```python
from build123d import *
from build123d.topology import SkipClean

# Parameters (mm, degrees)
EXTRUDE_1_DEPTH          = 48.25
EXTRUDE_1_DEPTH_BACK     = 48.25
EXTRUDE_2_DEPTH          = 3.75
EXTRUDE_2_DEPTH_BACK     = 3.75
SKETCH_2_R               = 7.5
SKETCH_2_R_2             = 5
CUT_EXTRUDE_1_DEPTH      = 3.75
CUT_EXTRUDE_1_DEPTH_BACK = 3.75
SKETCH_3_R               = 5
EXTRUDE_3_DEPTH          = 11.5
EXTRUDE_3_DEPTH_BACK     = 3.75
SKETCH_4_R               = 10
CUT_EXTRUDE_4_DEPTH      = 2
SKETCH_9_R               = 7.5
CUT_EXTRUDE_5_DEPTH      = 5
EXTRUDE_START            = 9
SKETCH_10_R              = 10
SKETCH_10_R_2            = 8.5
EXTRUDE_5_DEPTH          = 9
SKETCH_11_R              = 2.95
CUT_EXTRUDE_6_DEPTH      = 2
SKETCH_12_R              = 5.5
CUT_EXTRUDE_7_DEPTH      = 6
CUT_EXTRUDE_START        = -6
SKETCH_13_R              = 2.95
CUT_EXTRUDE_8_DEPTH      = 6


with BuildPart() as part:
    # Sketch 1 → Extrude 1 (new, two sides: drawn at the far end of the back side and taken through both)
    with BuildSketch(Plane(origin=(0, 0, 0), x_dir=(0, 0, -1), z_dir=(1, 0, 0)).offset(-EXTRUDE_1_DEPTH_BACK)):
        Polygon((3.75, 0), (3.75, 7.5), (-3.75, 7.5), (-3.75, -7.5), (3.75, -7.5), align=None)
    extrude(amount=EXTRUDE_1_DEPTH + EXTRUDE_1_DEPTH_BACK)

    # Sketch 2 → Extrude 2 (add, two sides: drawn at the far end of the back side and taken through both)
    with BuildSketch(Plane.XY.offset(-EXTRUDE_2_DEPTH_BACK)):
        with Locations((-48.25, 0)):
            Circle(SKETCH_2_R)
        with Locations((-48.25, 0)):
            Circle(SKETCH_2_R_2, mode=Mode.SUBTRACT)
    extrude(amount=EXTRUDE_2_DEPTH + EXTRUDE_2_DEPTH_BACK)

    # Sketch 3 → Cut-Extrude 1 (cut, two sides: drawn at the far end of the back side and taken through both)
    with BuildSketch(Plane.XY.offset(-CUT_EXTRUDE_1_DEPTH_BACK)):
        with Locations((-48.25, 0)):
            Circle(SKETCH_3_R)
    extrude(amount=CUT_EXTRUDE_1_DEPTH + CUT_EXTRUDE_1_DEPTH_BACK, mode=Mode.SUBTRACT)

    # Sketch 4 → Extrude 3 (add, two sides: drawn at the far end of the back side and taken through both)
    with BuildSketch(Plane.XY.offset(-EXTRUDE_3_DEPTH_BACK)):
        with Locations((48.25, 0)):
            Circle(SKETCH_4_R)
    extrude(amount=EXTRUDE_3_DEPTH + EXTRUDE_3_DEPTH_BACK)

    # Sketch 8 → Cut-Extrude 4 (cut)
    with BuildSketch(Plane.XY.offset(3.75)):
        with BuildLine():
            Line((0, 4.5), (-42.25, 4.5))
            ThreePointArc((-42.25, 4.5), (-40.75, 0), (-42.25, -4.5))
            Line((-42.25, -4.5), (0, -4.5))
            Line((0, -4.5), (39.31971445, -4.5))
            ThreePointArc((39.31971445, -4.5), (38.25, 0), (39.31971445, 4.5))
            Line((39.31971445, 4.5), (0, 4.5))
        make_face()
    extrude(amount=-CUT_EXTRUDE_4_DEPTH, mode=Mode.SUBTRACT)

    # Sketch 9 → Cut-Extrude 5 (cut)
    with BuildSketch(Plane.XY.offset(11.5)):
        with Locations((48.25, 0)):
            Circle(SKETCH_9_R)
    extrude(amount=-CUT_EXTRUDE_5_DEPTH, mode=Mode.SUBTRACT)

    # Sketch 10 → Extrude 5 (add)
    with SkipClean():  # the faces are left unmerged after this step: merging them gives an invalid solid
        with BuildSketch(Plane.XY.offset(11.5).offset(EXTRUDE_START)):
            with Locations((48.25, 0)):
                Circle(SKETCH_10_R)
            with Locations((48.25, 0)):
                Circle(SKETCH_10_R_2, mode=Mode.SUBTRACT)
        extrude(amount=-EXTRUDE_5_DEPTH)

    # Sketch 11 → Cut-Extrude 6 (cut)
    with SkipClean():  # the faces are left unmerged after this step: merging them gives an invalid solid
        with BuildSketch(Plane.XY.offset(6.5)):
            with Locations((48.25, 0)):
                Circle(SKETCH_11_R)
        extrude(amount=-CUT_EXTRUDE_6_DEPTH, mode=Mode.SUBTRACT)

    # Sketch 12 → Cut-Extrude 7 (cut)
    with SkipClean():  # the faces are left unmerged after this step: merging them gives an invalid solid
        with BuildSketch(Plane(origin=(0, 0, -3.75), x_dir=(-1, 0, 0), z_dir=(0, 0, -1))):
            with Locations((-48.25, 0)):
                Circle(SKETCH_12_R)
        extrude(amount=-CUT_EXTRUDE_7_DEPTH, mode=Mode.SUBTRACT)

    # Sketch 13 → Cut-Extrude 8 (cut)
    with SkipClean():  # the faces are left unmerged after this step: merging them gives an invalid solid
        with BuildSketch(Plane(origin=(0, 0, 2.25), x_dir=(-1, 0, 0), z_dir=(0, 0, -1)).offset(CUT_EXTRUDE_START)):
            with Locations(Location((-48.25, 0, 0), (0, 0, 180))):
                Circle(SKETCH_13_R)
        extrude(amount=CUT_EXTRUDE_8_DEPTH, mode=Mode.SUBTRACT)


solid = part.part
```
Could you check a few things on this model? Use its own coordinates, in mm. A direction names the side the tool comes from. Give positions to 0.01 mm unless a question says otherwise; leave off trailing zeros. Loops run counter-clockwise (first coordinate to the right, second up) from the corner with the lowest first, then second, coordinate; pieces in that order, holes last. Notation, with made-up numbers: (80.25, 62) - (124.25, 62) arc R25 cw to (124.25, 79) - close; hole circle Ø3 at (19, 46). An arc over 180 degrees is marked (long way). Use one line per item in the form item = value.
1. I want a section at B-B (z = 15.5). Please give me the cut outline in (x, y).
Response values:
outline = circle Ø20 at (48.25, 0); hole circle Ø17 at (48.25, 0)
2. Thinking about a two-plate mould opening in X: for faces 4 (the face through (45.2, -8.1, 20.5)), 5 (the face through (-55.75, 0.16, -0.05)), 6 (the face through (48.1, -3.2, 6.5)), which applies, released by +X, released by -X, zero draft, split by the parting line, or undercut?
Response values:
face_4 = zero draft
face_5 = released by -X
face_6 = undercut
3. I'm going to push flat-ended pins straight in: pin 1 Ø1.6 at (x, z) = (9.5, 3) entering from +Y; pin 2 Ø0.6 at (x, z) = (-19.5, 3) entering from -Y; pin 3 Ø12 at (x, y) = (0, -3) entering from +Z. Where does each tip first touch, or does it pass through?
Response values:
pin_1 = 7.5
pin_2 = -7.5
pin_3 = 3.75
4. On a 3-axis mill with a long thin cutter (end or side, diameter ignored), from which of +Z, -Z, +X, -X, +Y, -Y can I reach the whole of each face in a straight line? I mean faces 1 (the face through (48, -8, 11.5)), 2 (the face through (-4, -7.5, 0)), 3 (the face through (53.745, 0.242, -0.792)). Say none if no direction works.
Response values:
face_1 = +Z
face_2 = +Z, -Z, -X, -Y
face_3 = -Z
5. I want a section at C-C (x = 16). Please give me the cut outline in (y, z), and give its area (3 significant figures).
Response values:
outline = (-7.5, -3.75) - (7.5, -3.75) - (7.5, 3.75) - (4.5, 3.75) - (4.5, 1.75) - (-4.5, 1.75) - (-4.5, 3.75) - (-7.5, 3.75) - close
area = 94.5 mm²
6. I need wall thicknesses on probe 1 along Y at (x, z) = (48.25, 3.4); probe 2 along Y at (x, z) = (48.25, 10); probe 3 along Z at (x, y) = (29, -3.5). Which ranges of each line are inside material? Lowest first, please.
Response values:
probe_1 = -10 to -2.95, 2.95 to 10
probe_2 = -10 to -7.5, 7.5 to 10
probe_3 = -3.75 to 1.75
